The model under review builds one solid part; all positions refer to its coordinate system, in mm. Face numbers are marked on the shaded views. Give positions to 0.01 mm unless a question says otherwise; leave off trailing zeros. Order: outer loops, then holes, each group sorted by start corner. A loop starts at its lowest first (then second) coordinate and runs counter-clockwise, first axis right, second up. Notation, with made-up numbers: (-20, 88) -> (10, 88) arc R7 ccw to (10, 92) -> close; hole circle Ø4 at (16, 15). An arc over 180 degrees is marked (long way). Use one line per item in the form item = value.
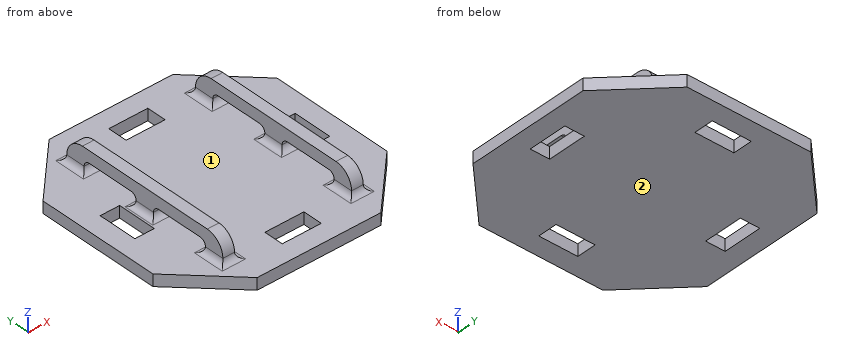
Autodesk Fusion 360 part; units mm, degrees
sketch "Sketch1" plane through (0, 0, 0) normal (0, 0, 1) x (1, 0, 0)
  line L0 (0, 0) -> (60, 0)
  line L1 (60, 0) -> (60, 60)
  line L2 (60, 60) -> (0, 60)
  line L3 (0, 60) -> (0, 0)
  line L4 (0, 45.8579) -> (14.1421, 60)
  line L5 (0, 45.8579) -> (19.799, 45.8579) construction
  line L6 (14.1421, 0) -> (0, 14.1421)
  line L7 (14.1421, 0) -> (24.1421, 0) construction
  line L8 (60, 14.1421) -> (45.8579, 0)
  line L9 (60, 14.1421) -> (83.1045, 14.1421) construction
  line L10 (45.8579, 60) -> (60, 45.8579)
  line L11 (0, 30) -> (60, 30) construction
  line L12 (30, 60) -> (30, 0) construction
  line L13 (25, 55) -> (35, 55)
  line L14 (35, 55) -> (35, 50)
  line L15 (35, 50) -> (25, 50)
  line L16 (25, 50) -> (25, 55)
  line L17 (5, 25) -> (5, 35)
  line L18 (10, 35) -> (10, 25)
  line L19 (10, 25) -> (5, 25)
  line L20 (5, 35) -> (10, 35)
  line L21 (35, 5) -> (25, 5)
  line L22 (25, 10) -> (35, 10)
  line L23 (35, 10) -> (35, 5)
  line L24 (25, 5) -> (25, 10)
  line L25 (55, 35) -> (55, 25)
  line L26 (50, 25) -> (50, 35)
  line L27 (50, 35) -> (55, 35)
  line L28 (55, 25) -> (50, 25)
  point P0 (30, 30)
  dimension "d1" = 60
  dimension "d2" = 60
  dimension "d3" = 45
  dimension "d4" = 135
  dimension "d5" = 135
  dimension "d6" = 90
  dimension "d7" = 20
  dimension "d8" = 10
  dimension "d9" = 5
  dimension "d10" = 5
  dimension "d11" = 20
  dimension "d13" = 360
extrude "Extrude1" add sketch "Sketch1" along normal blind 3 contours L0 L1 L2 L3 L4 L6 L8 L10
sketch "Sketch2" plane through (0, 0, 3) normal (0, 0, 1) x (-1, 0, 0)
  line L0 (-5, -25) -> (-5, -35)
  line L1 (-5, -35) -> (-10, -35)
  line L2 (-10, -35) -> (-10, -25)
  line L3 (-10, -25) -> (-5, -25)
  line L4 (-55, -35) -> (-55, -25)
  line L5 (-55, -25) -> (-50, -25)
  line L6 (-50, -25) -> (-50, -35)
  line L7 (-50, -35) -> (-55, -35)
  line L8 (-35, -5) -> (-25, -5)
  line L9 (-25, -5) -> (-25, -10)
  line L10 (-25, -10) -> (-35, -10)
  line L11 (-35, -10) -> (-35, -5)
  line L12 (-35, -50) -> (-25, -50)
  line L13 (-25, -50) -> (-25, -55)
  line L14 (-25, -55) -> (-35, -55)
  line L15 (-35, -55) -> (-35, -50)
  line L16 (0, -45.8579) -> (0, -14.1421)
  line L17 (0, -14.1421) -> (-14.1421, 0)
  line L18 (-14.1421, 0) -> (-45.8579, 0)
  line L19 (-45.8579, 0) -> (-60, -14.1421)
  line L20 (-60, -14.1421) -> (-60, -45.8579)
  line L21 (-60, -45.8579) -> (-45.8579, -60)
  line L22 (-45.8579, -60) -> (-14.1421, -60)
  line L23 (-14.1421, -60) -> (0, -45.8579)
ref_plane "WorkPlane1" through (30, 0, 0) normal (1, 0, 0) x (0, 1, 0)
sketch "Sketch3" plane through (30, 0, 0) normal (1, 0, 0) x (0, 1, 0)
  line L0 (52.5, 3) -> (7.5, 3)
  line L1 (7.5, 3) -> (7.5, 9)
  line L2 (7.5, 9) -> (52.5, 9)
  line L3 (52.5, 9) -> (52.5, 3)
  line L4 (47.5, 3) -> (32.5, 3)
  line L5 (32.5, 3) -> (32.5, 6)
  line L6 (32.5, 6) -> (47.5, 6)
  line L7 (47.5, 6) -> (47.5, 3)
  line L8 (27.5, 3) -> (12.5, 3)
  line L9 (12.5, 3) -> (12.5, 6)
  line L10 (12.5, 6) -> (27.5, 6)
  line L11 (27.5, 6) -> (27.5, 3)
  line L12 (60, 3) -> (0, 3)
  line L13 (0, 3) -> (0, 0)
  line L14 (0, 0) -> (60, 0)
  line L15 (60, 0) -> (60, 3)
  point P0 (30, 0)
  dimension "d17" = 45
  dimension "d18" = 6
  dimension "d21" = 3
  dimension "d22" = 5
  dimension "d23" = 5
  dimension "d24" = 5
  dimension "d25" = 22.5
extrude "Extrude2" add sketch "Sketch3" along normal blind 3 from surface at 15 contours L0 L1 L2 L3 L5 L6 L7 L9 L10 L11 L12
extrude "Extrude3" add sketch "Sketch3" against normal blind 3 from surface at -15 contours L0 L1 L2 L3 L5 L6 L7 L9 L10 L11 L12
fillet "Fillet1" radius 1.5 24 edges at (13.5, 27.5, 3) (15, 30, 3) (13.5, 47.5, 3) (15, 50, 3) (13.5, 7.5, 3) (15, 10, 3) (46.5, 7.5, 3) (48, 10, 3) (46.5, 27.5, 3) (48, 30, 3) (46.5, 47.5, 3) (48, 50, 3) (46.5, 52.5, 3) (45, 50, 3) (46.5, 32.5, 3) (45, 30, 3) (46.5, 12.5, 3) (45, 10, 3) (13.5, 52.5, 3) (12, 50, 3) (13.5, 32.5, 3) (12, 30, 3) (13.5, 12.5, 3) (12, 10, 3)
fillet "Fillet1" radius 1.5 8 edges at (13.5, 12.5, 6) (13.5, 47.5, 6) (46.5, 27.5, 6) (46.5, 47.5, 6) (13.5, 27.5, 6) (13.5, 32.5, 6) (46.5, 32.5, 6) (46.5, 12.5, 6)
fillet "Fillet1" radius 4.5 4 edges at (13.5, 52.5, 9) (13.5, 7.5, 9) (46.5, 7.5, 9) (46.5, 52.5, 9)
equation "d1 = d2"
equation "d9 = d8 / 2"
equation "d23 = d22"
equation "d24 = d22"
equation "d25 = d17 / 2"
1. Add section D-D on y = 29.5. Give the boundary of the cut face in (x, z).
Values:
outline = (0, 0) -> (5, 0) -> (5, 3) -> (0, 3) -> close; (10, 0) -> (50, 0) -> (50, 3) -> (49.5, 3) arc R1.5 cw to (48, 4.5) -> (48, 9) -> (45, 9) -> (45, 4.5) arc R1.5 cw to (43.5, 3) -> (16.5, 3) arc R1.5 cw to (15, 4.5) -> (15, 9) -> (12, 9) -> (12, 4.5) arc R1.5 cw to (10.5, 3) -> (10, 3) -> close; (55, 0) -> (60, 0) -> (60, 3) -> (55, 3) -> close
2. Add section B-B on x = 27.5. Give the boundary of the cut face in (y, z), then the cut area to 3 significant figures.
Values:
outline = (0, 0) -> (5, 0) -> (5, 3) -> (0, 3) -> close; (10, 0) -> (50, 0) -> (50, 3) -> (10, 3) -> close; (55, 0) -> (60, 0) -> (60, 3) -> (55, 3) -> close
area = 150 mm^2
3. Add section A-A on y = 17. Give the boundary of the cut face in (x, z), then the cut area to 3 significant figures.
Values:
outline = (0, 0) -> (60, 0) -> (60, 3) -> (0, 3) -> close; (12, 6) -> (15, 6) -> (15, 9) -> (12, 9) -> close; (45, 6) -> (48, 6) -> (48, 9) -> (45, 9) -> close
area = 198 mm^2
4. For L1, parallel to Y at x = 27.5, z = 0.75; L2, parallel to X at y = 11, z = 5.25; L3, parallel to Z at x = 23, y = 32, list the stretches that pass through material, from the lowest coordinate up.
Values:
L1 = 0 to 5, 10 to 50, 55 to 60
L2 = 12 to 15, 45 to 48
L3 = 0 to 3
5. The part is to be moulded in two halves that separate along X. For the marked faces 1 and 2, say which applies: +X half, -X half, draft (parallel to the pull), parting line (faces both ways), or undercut.
Values:
face_1 = undercut
face_2 = draft
6. For pin 1 Ø1.5 at (x, y) = (20.5, 23.5) entering from +Z; pin 2 Ø4 at (x, z) = (14.5, 6.5) entering from +Y; pin 3 Ø4 at (y, z) = (53.5, 1.5) entering from -X, all flat-tipped, find the tip position at first contact; note any pin that passes through.
Values:
pin_1 = 3
pin_2 = 52.5
pin_3 = 5.64
7. Add section C-C on z = 6.75. Give the boundary of the cut face in (x, y), then the cut area to 3 significant figures.
Values:
outline = (12, 8.1) -> (15, 8.1) -> (15, 51.9) -> (12, 51.9) -> close; (45, 8.1) -> (48, 8.1) -> (48, 51.9) -> (45, 51.9) -> close
area = 263 mm^2
